Autodesk Inventor part; units mm, degrees
ref_plane "YZ Plane" through (0, 0, 0) normal (1, 0, 0) x (0, 1, 0)
ref_plane "XZ Plane" through (0, 0, 0) normal (0, 1, 0) x (-1, 0, 0)
ref_plane "XY Plane" through (0, 0, 0) normal (0, 0, 1) x (1, 0, 0)
sketch "Skizze1" plane through (0, 0, 0) normal (0, 1, 0) x (-1, 0, 0)
  line L0 (-10, -50) -> (10, -50)
  line L1 (10, -50) -> (10, 50)
  line L2 (10, 50) -> (-10, 50)
  line L3 (-10, 50) -> (-10, -50)
  line L4 (-10, -50) -> (10, 50) construction
  line L5 (10, -50) -> (-10, 50) construction
  point P0 (0, 0)
  dimension "d0" = 20
  dimension "d1" = 100
extrude "Extrusion1" add sketch "Skizze1" along normal blind 4
fillet "Rundung1" radius 10 4 edges at (10, 2, -50) (-10, 2, -50) (10, 2, 50) (-10, 2, 50)
sketch "Skizze2" plane through (0, 0, 0) normal (0, -1, 0) x (1, 0, 0)
  point P0 (0, 0)
sketch "Skizze3" plane through (0, 0, 0) normal (0, -1, 0) x (1, 0, 0)
  line L0 (-17.5, 34) -> (-17.5, 46)
  line L1 (17.5, 46) -> (17.5, 34)
  line L2 (-11.5, 46) -> (-11.5, 34)
  line L3 (11.5, 46) -> (11.5, 34)
  line L4 (0, -70) -> (0, 70)
  line L5 (-17.5, 46) -> (-11.5, 46)
  line L6 (11.5, 46) -> (17.5, 46)
  line L7 (17.5, 34) -> (11.5, 34)
  line L8 (-11.5, 34) -> (-17.5, 34)
  point P0 (0, 0)
  point P1 (0, 34)
  point P2 (11.5, 40)
  point P3 (17.5, 40)
  point P4 (-11.5, 40)
  point P5 (-17.5, 40)
  point P6 (14.5, 34)
  point P7 (-14.5, 34)
  dimension "d6" = 12
  dimension "d7" = 35
  dimension "d11" = 23
  dimension "d12" = 34
  dimension "d13" = 6
sketch "Skizze4" plane through (0, 0, 0) normal (0, -1, 0) x (1, 0, 0)
  arc A0 (10, 40) -> (-10, 40) centre (0, 40) ccw
  line L0 (-11.5, 34) -> (-17.5, 34)
  line L1 (11.5, 46) -> (11.5, 34)
  line L2 (-11.5, 34) -> (11.5, 34)
  line L3 (11.5, 34) -> (11.5, 53)
  line L4 (11.5, 53) -> (-11.5, 53)
  line L5 (-11.5, 53) -> (-11.5, 34)
  point P0 (0, 0)
  dimension "d14" = 19
extrude "Extrusion2" cut sketch "Skizze4" against normal blind 4
extrude "Extrusion3" add sketch "Skizze3" along normal blind 2 and the other way blind 5
sketch "Skizze5" plane through (0, 0, 0) normal (0, -1, 0) x (1, 0, 0)
  line L0 (-17.5, 34) -> (-11.5, 34)
  line L1 (11.5, 34) -> (17.5, 34)
  line L2 (-17.5, 34) -> (17.5, 34)
  line L3 (17.5, 34) -> (17.5, 32)
  line L4 (17.5, 32) -> (-17.5, 32)
  line L5 (-17.5, 32) -> (-17.5, 34)
  point P0 (0, 0)
  dimension "d21" = 2
extrude "Extrusion4" add sketch "Skizze5" along normal blind 2 and the other way blind 21
fillet "Rundung2" radius 1 4 edges at (10, 2, 32) (0, 0, 32) (0, 4, 32) (-10, 2, 32)
chamfer "Fasen1" distance 0.4 angle 45 7 edges at (-11.5, -2, 40) (-11.5, 1.5, 46) (11.5, -2, 40) (11.5, 1.5, 46) (-11.5, 5, 40) (11.5, 5, 40) (0, -2, 34)
fillet "Rundung3" radius 0.4 19 edges at (-14.7, -2, 46) (-14.7, 5, 46) (-17.5, 1.5, 46) (14.7, 5, 46) (14.7, -2, 46) (17.5, 1.5, 46) (17.5, -2, 39) (17.5, 5, 40) (17.5, 13, 34) (17.5, 9.5, 32) (0, 21, 34) (0, -2, 32) (-17.5, 13, 34) (-17.5, 21, 33) (-17.5, 9.5, 32) (-17.5, -2, 39) (-17.5, 5, 40) (17.5, 21, 33) (0, 21, 32)
sketch "Skizze6" plane through (0, -2, 0) normal (0, -1, 0) x (1, 0, 0)
  line L0 (-17.1, 45.6) -> (-11.9, 45.6)
  line L1 (11.9, 45.6) -> (17.1, 45.6)
  line L2 (11.5, 34) -> (-11.5, 34)
  line L3 (0, -69.2) -> (0, 65.2)
  point P0 (0, 0)
  point P1 (-13.5, 40)
  point P2 (13.5, 40)
  dimension "d31" = 6
  dimension "d32" = 27
hole "Bohrung1" at (-13.5, -2, 40) at (13.5, -2, 40) direction (0, 1, 0) diameter 1 end through all
properties part number "L1"
The model under review builds one solid part; all positions refer to its coordinate system, in mm. A direction names the side the tool comes from. Round coordinates to 2 decimals unless told otherwise and drop trailing zeros. Loops run counter-clockwise (first coordinate to the right, second up) from the corner with the lowest first, then second, coordinate; pieces in that order, holes last. Notation, with made-up numbers: (-13.75, 87) - (32.25, 87) arc R21 cw to (32.25, 113) - close; hole circle Ø9 at (-16.5, -25). An arc over 180 degrees is marked (long way). Write each question's results on one line, items separated by ' | '. Start each with the question number.
Q1. Take a section at D-D on x = -4. Give the boundary of the cut face in (y, z), plus the area to 3 significant figures.
Q2. Take a section at C-C on z = 2. Give the boundary of the cut face in (x, y), plus the area to 3 significant figures.
Q3. Tool access review of faces 1 (the flat face through (-10, 2, -5)), 2 (the flat face through (0, 0, -9)), 3 (the flat face through (10, 2, -4)), 4 (the flat face through (0, 4, -9)), 5 (the flat face through (-11.5, 2, 40)): name each direction out of +Z, -Z, +X, -X, +Y, -Y from which nothing blocks a thin tool from reaching the whole face with its end or side.
Q4. Insertion check: P1, Ø3, axis at x = 4, y = 7, coming from the +Z side; P2, Ø10, axis at x = 12.5, z = -18.5, coming from the +Y side; P3, Ø1.5, axis at x = -9, z = -40, coming from the -Y side. Each pin has a flat end and moves straight along its axis. Give the tip position at first contact, or say it passes through.
Q5. Take a section at B-B on y = 16. Give the boundary of the cut face in (x, z).
Q6. Wall thickness on line 1 along X through (y, z) = (3, 40); line 2 along Z through (x, y) = (-13.5, 3); line 3 along Y through (x, z) = (-3, 17): over which ranges is each line inside the solid? List them lowest first. Write a range as [from, to].
Q7. Take a section at A-A on x = 15.5. Give the boundary of the cut face in (y, z).
Data:
1) outline: (-2, 32.4) arc R0.4 ccw to (-1.6, 32) - (-1, 32) arc R1 cw to (0, 31) - (0, -49.17) - (4, -49.17) - (4, 31) arc R1 cw to (5, 32) - (20.6, 32) arc R0.4 ccw to (21, 32.4) - (21, 33.6) arc R0.4 ccw to (20.6, 34) - (-1.6, 34) - (-2, 33.6) - close | area: 371 mm²
2) outline: (-10, 0) - (10, 0) - (10, 4) - (-10, 4) - close | area: 80.0 mm²
3) face 1: -Z, -X, +Y, -Y | face 2: -Z, +X, -X, -Y | face 3: -Z, +X, +Y, -Y | face 4: -Z, +X, -X, +Y | face 5: +Z, +Y, -Y
4) P1: stops at z = 34 | P2: stops at y = 4 | P3: stops at y = 0
5) outline: (-17.5, 32.4) arc R0.4 ccw to (-17.1, 32) - (17.1, 32) arc R0.4 ccw to (17.5, 32.4) - (17.5, 33.6) arc R0.4 ccw to (17.1, 34) - (-17.1, 34) arc R0.4 ccw to (-17.5, 33.6) - close
6) line 1: x = [-17.5, -14], [-13, -11.5], [11.5, 13], [14, 17.5] | line 2: z = [32, 39.5], [40.5, 46] | line 3: y = [0, 4]
7) outline: (-2, 32.4) arc R0.4 ccw to (-1.6, 32) - (20.6, 32) arc R0.4 ccw to (21, 32.4) - (21, 33.6) arc R0.4 ccw to (20.6, 34) - (5, 34) - (5, 45.6) arc R0.4 ccw to (4.6, 46) - (-1.6, 46) arc R0.4 ccw to (-2, 45.6) - close
